from build123d import *

# Parameters (mm, degrees)
BOSS_EXTRUDE1_DEPTH = 5
SKETCH2_R           = 7
BOSS_EXTRUDE2_DEPTH = 65
SKETCH3_R           = 4
CUT_EXTRUDE1_DEPTH  = 20


with BuildPart() as part:
    # Sketch1 → Boss-Extrude1 (new body)
    with BuildSketch(Plane.XY):
        Polygon((8.660254038, -5), (8.660254038, 5), (0, 10), (-8.660254038, 5), (-8.660254038, -5), (0, -10), align=None)
    extrude(amount=BOSS_EXTRUDE1_DEPTH)

    # Sketch2 → Boss-Extrude2 (add)
    with BuildSketch(Plane.XY.offset(5)):
        Circle(SKETCH2_R)
    extrude(amount=BOSS_EXTRUDE2_DEPTH)

    # Sketch3 → Cut-Extrude1 (cut)
    with BuildSketch(Plane.XY.offset(70)):
        Circle(SKETCH3_R)
    extrude(amount=-CUT_EXTRUDE1_DEPTH, mode=Mode.SUBTRACT)


solid = part.part
Input: part model. Units: mm. Frame: model coordinates. A direction names the side the tool comes from. Round coordinates to 2 decimals unless told otherwise and drop trailing zeros. Loops run counter-clockwise (first coordinate to the right, second up) from the corner with the lowest first, then second, coordinate; pieces in that order, holes last. Notation, with made-up numbers: (-37.75, 52.5) -> (-2.75, 52.5) arc R10 cw to (-2.75, 64.5) -> close; hole circle Ø3 at (37.25, 56). An arc over 180 degrees is marked (long way). Answer as a JSON object with one key per item and string values. Group by question number.
1) Section query B-B on z = 51.5. Output: boundary loops of the cut face in (x, y).
2) Pin query (flat end, axial travel): pin 1 (1.5 mm diameter, centred on x = -6, z = 22, fed in from -Y); pin 2 (2.5 mm diameter, centred on x = 1.5, y = -1, fed in from +Z); pin 3 (6 mm diameter, centred on x = -1, z = 38.5, fed in from -Y). Return the tip coordinate at first contact, or that it passes through.
3) Section query D-D on y = 8. Output: boundary loops of the cut face in (x, z).
4) Section query C-C on z = 36. Output: boundary loops of the cut face in (x, y), plus the area to 3 significant figures.
5) Ray query, L1, parallel to Y at x = 0, z = 56.75; L2, parallel to Z at x = 0, y = -0.75; L3, parallel to Z at x = 6, y = -5.75. Return the intervals inside material, ascending.
6) Section query A-A on y = 0. Output: boundary loops of the cut face in (x, z).
7) Reachability of faces 4 (the cylindrical face through (6.466, -2.681, 37.045)), 5 (the flat face through (-4.391, -7.465, 2.465)) from +Z, -Z, +X, -X, +Y, -Y: full face, straight path, thin tool, end or side. Return the list, or none.
8) Draft query along X for faces 1 (the flat face through (0, 0, 50)), 2 (the flat face through (-8.66, 0, 2)), 3 (the flat face through (4.27, -7.535, 2.465)). Return one class per face: +X half, -X half, draft (parallel to the pull), parting line (faces both ways), or undercut.
Reply:
{
 "1": {"outline": "circle Ø14 at (0, 0); hole circle Ø8 at (0, 0)"},
 "2": {"pin 1": "stops at y = -4.63", "pin 2": "stops at z = 50", "pin 3": "stops at y = -7"},
 "3": {"outline": "(-3.46, 0) -> (3.46, 0) -> (3.46, 5) -> (-3.46, 5) -> close"},
 "4": {"outline": "circle Ø14 at (0, 0)", "area": "154 mm2"},
 "5": {"L1": "y = -7 to -4, 4 to 7", "L2": "z = 0 to 50", "L3": "z = 0 to 5"},
 "6": {"outline": "(-8.66, 0) -> (8.66, 0) -> (8.66, 5) -> (7, 5) -> (7, 70) -> (4, 70) -> (4, 50) -> (-4, 50) -> (-4, 70) -> (-7, 70) -> (-7, 5) -> (-8.66, 5) -> close"},
 "7": {"face 4": "+Z", "face 5": "+Z, -Z, -X, -Y"},
 "8": {"face 1": "undercut", "face 2": "-X half", "face 3": "+X half"}
}
